CAD build for the part. Positions are in the model's coordinates, mm. A direction names the side the tool comes from. Round coordinates to 2 decimals unless told otherwise and drop trailing zeros. Put each result on its own line as item: value. Start each with the question number.
from build123d import *

# Parameters (mm, degrees)
F0_W     = 84
F0_H     = 60
F1_DEPTH = 4
F2_W     = 4
F2_H     = 4
F3_DEPTH = 4
F5_DEPTH = 4


with BuildPart() as f1:
    # F0 (on Top) → F1 (new body)
    with BuildSketch(Plane.XY):
        with Locations((42, 30)):
            Rectangle(F0_W, F0_H)
    extrude(amount=F1_DEPTH)

    # F2 (on face) → F3 (cut, through all)
    with BuildSketch(Plane.XY.offset(4)):
        with Locations((2, 2)):
            Rectangle(F2_W, F2_H)
        with Locations((2, 58)):
            Rectangle(F2_W, F2_H)
        with Locations((82, 2)):
            Rectangle(F2_W, F2_H)
        with Locations((82, 58)):
            Rectangle(F2_W, F2_H)
    extrude(amount=-F3_DEPTH, mode=Mode.SUBTRACT)

    # F4 (on face) → F5 (cut, through all)
    with BuildSketch(Plane.XY.offset(4)):
        with BuildLine():
            ThreePointArc((10.5, 50), (9.792893, 49.707107), (9.5, 49))
            Line((9.5, 49), (9.5, 11))
            ThreePointArc((9.5, 11), (9.792893, 10.292893), (10.5, 10))
            ThreePointArc((10.5, 10), (11.207107, 10.292893), (11.5, 11))
            Line((11.5, 11), (11.5, 49))
            ThreePointArc((11.5, 49), (11.207107, 49.707107), (10.5, 50))
        make_face()
        with BuildLine():
            ThreePointArc((17.5, 50), (16.792893, 49.707107), (16.5, 49))
            Line((16.5, 49), (16.5, 11))
            ThreePointArc((16.5, 11), (16.792893, 10.292893), (17.5, 10))
            ThreePointArc((17.5, 10), (18.207107, 10.292893), (18.5, 11))
            Line((18.5, 11), (18.5, 49))
            ThreePointArc((18.5, 49), (18.207107, 49.707107), (17.5, 50))
        make_face()
        with BuildLine():
            ThreePointArc((24.5, 50), (23.792893, 49.707107), (23.5, 49))
            Line((23.5, 49), (23.5, 11))
            ThreePointArc((23.5, 11), (23.792893, 10.292893), (24.5, 10))
            ThreePointArc((24.5, 10), (25.207107, 10.292893), (25.5, 11))
            Line((25.5, 11), (25.5, 49))
            ThreePointArc((25.5, 49), (25.207107, 49.707107), (24.5, 50))
        make_face()
        with BuildLine():
            ThreePointArc((31.5, 50), (30.792893, 49.707107), (30.5, 49))
            Line((30.5, 49), (30.5, 11))
            ThreePointArc((30.5, 11), (30.792893, 10.292893), (31.5, 10))
            ThreePointArc((31.5, 10), (32.207107, 10.292893), (32.5, 11))
            Line((32.5, 11), (32.5, 49))
            ThreePointArc((32.5, 49), (32.207107, 49.707107), (31.5, 50))
        make_face()
        with BuildLine():
            ThreePointArc((38.5, 50), (37.792893, 49.707107), (37.5, 49))
            Line((37.5, 49), (37.5, 11))
            ThreePointArc((37.5, 11), (37.792893, 10.292893), (38.5, 10))
            ThreePointArc((38.5, 10), (39.207107, 10.292893), (39.5, 11))
            Line((39.5, 11), (39.5, 49))
            ThreePointArc((39.5, 49), (39.207107, 49.707107), (38.5, 50))
        make_face()
        with BuildLine():
            ThreePointArc((45.5, 50), (44.792893, 49.707107), (44.5, 49))
            Line((44.5, 49), (44.5, 11))
            ThreePointArc((44.5, 11), (44.792893, 10.292893), (45.5, 10))
            ThreePointArc((45.5, 10), (46.207107, 10.292893), (46.5, 11))
            Line((46.5, 11), (46.5, 49))
            ThreePointArc((46.5, 49), (46.207107, 49.707107), (45.5, 50))
        make_face()
        with BuildLine():
            ThreePointArc((52.5, 50), (51.792893, 49.707107), (51.5, 49))
            Line((51.5, 49), (51.5, 11))
            ThreePointArc((51.5, 11), (51.792893, 10.292893), (52.5, 10))
            ThreePointArc((52.5, 10), (53.207107, 10.292893), (53.5, 11))
            Line((53.5, 11), (53.5, 49))
            ThreePointArc((53.5, 49), (53.207107, 49.707107), (52.5, 50))
        make_face()
        with BuildLine():
            ThreePointArc((59.5, 50), (58.792893, 49.707107), (58.5, 49))
            Line((58.5, 49), (58.5, 11))
            ThreePointArc((58.5, 11), (58.792893, 10.292893), (59.5, 10))
            ThreePointArc((59.5, 10), (60.207107, 10.292893), (60.5, 11))
            Line((60.5, 11), (60.5, 49))
            ThreePointArc((60.5, 49), (60.207107, 49.707107), (59.5, 50))
        make_face()
        with BuildLine():
            ThreePointArc((66.5, 50), (65.792893, 49.707107), (65.5, 49))
            Line((65.5, 49), (65.5, 11))
            ThreePointArc((65.5, 11), (65.792893, 10.292893), (66.5, 10))
            ThreePointArc((66.5, 10), (67.207107, 10.292893), (67.5, 11))
            Line((67.5, 11), (67.5, 49))
            ThreePointArc((67.5, 49), (67.207107, 49.707107), (66.5, 50))
        make_face()
        with BuildLine():
            ThreePointArc((73.5, 50), (72.792893, 49.707107), (72.5, 49))
            Line((72.5, 49), (72.5, 11))
            ThreePointArc((72.5, 11), (72.792893, 10.292893), (73.5, 10))
            ThreePointArc((73.5, 10), (74.207107, 10.292893), (74.5, 11))
            Line((74.5, 11), (74.5, 49))
            ThreePointArc((74.5, 49), (74.207107, 49.707107), (73.5, 50))
        make_face()
    extrude(amount=-F5_DEPTH, mode=Mode.SUBTRACT)


solid = f1.part
(1) Tool access for faces 4 (the flat face through (41, 30, 4)), 5 (the flat face through (41, 0, 2)), 6 (the flat face through (58.5, 30, 2)), 7 (the flat face through (80, 2, 2)), 8 (the flat face through (4, 2, 2)): list every direction of +Z, -Z, +X, -X, +Y, -Y with a clear straight run to the whole face (end or side of a thin tool).
(2) Drill centre lines: line 1 along Y through (x, z) = (10.5, 1.25); line 2 along X through (y, z) = (57, 2.85); line 3 along Y through (x, z) = (45, 0.95). Where is each one in solid material? Low to high.
(3) Cut at A-A on y = 46. Count the separate pieces of the cut face and the enclosed holes in it, and give its area (3 significant figures).
(4) Mould opens along Y. For faces 1 (the flat face through (30.5, 30, 2)), 2 (the flat face through (2, 4, 2)), 3 (the flat face through (41, 30, 0)) say: +Y half, -Y half, draft (parallel to the pull), parting line (faces both ways), or undercut.
(5) Flat gauge pin, fed straight in: pin 1 Ø2 at (x, z) = (2.5, 2.5) entering from +Y. Where does the tip first touch, or does it go through?
Taken from the geometry:
1. face 4: +Z, +X, -X, +Y, -Y
1. face 5: +Z, -Z, +X, -X, -Y
1. face 6: +Z, -Z
1. face 7: +Z, -Z, +X, -Y
1. face 8: +Z, -Z, -X, -Y
2. line 1: 0 to 10, 50 to 60
2. line 2: 4 to 80
2. line 3: 0 to 10.13, 49.87 to 60
3. separate pieces: 11
3. enclosed holes: 0
3. area: 256 mm2
4. face 1: undercut
4. face 2: -Y half
4. face 3: draft
5. pin 1: y = 56
